Design review of the part shown in the three views and the two pictorial views. Dimensions are in mm from the part's minimum x, y and z. Give positions to 0.01 mm unless a question says otherwise; leave off trailing zeros. Loops run counter-clockwise (first coordinate to the right, second up) from the corner with the lowest first, then second, coordinate; pieces in that order, holes last. Notation, with made-up numbers: (-14.75, 44.25) -> (21.25, 44.25) arc R32 ccw to (21.25, 75.25) -> close; hole circle Ø9 at (-0.75, 79.25). An arc over 180 degrees is marked (long way). Answer as CSV lines item,"result".
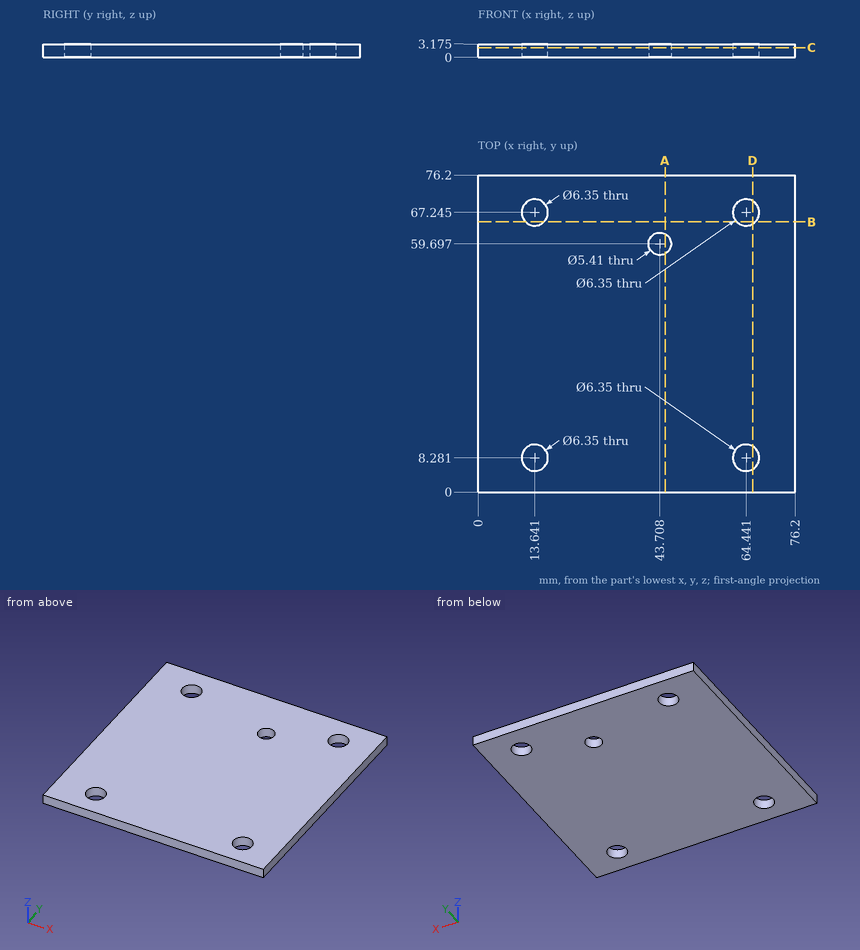
Q1. We need section D-D, the plane x = 66. State the section outline as (y, z) points (1 decimal).
Filled sheet:
outline,"(0, 0) -> (5.5, 0) -> (5.5, 3.2) -> (0, 3.2) -> close; (11, 0) -> (64.5, 0) -> (64.5, 3.2) -> (11, 3.2) -> close; (70, 0) -> (76.2, 0) -> (76.2, 3.2) -> (70, 3.2) -> close"
Q2. To check wall thickness, follow probe 1 along X at (y, z) = (67, 1.7) (1 decimal); probe 2 along Y at (x, z) = (67, 1.45) (1 decimal); probe 3 along X at (y, z) = (5.5, 2.8) (1 decimal). State the ranges of each line that lie inside material, in increasing order. Write a range as from..to.
Filled sheet:
probe 1,"x = 0..10.5, 16.8..61.3, 67.6..76.2"
probe 2,"y = 0..6.4, 10.2..65.4, 69.1..76.2"
probe 3,"x = 0..12.1, 15.2..62.9, 66..76.2"
Q3. We need section B-B, the plane y = 65. State the section outline as (x, z) points (1 decimal).
Filled sheet:
outline,"(0, 0) -> (11.4, 0) -> (11.4, 3.2) -> (0, 3.2) -> close; (15.9, 0) -> (62.2, 0) -> (62.2, 3.2) -> (15.9, 3.2) -> close; (66.7, 0) -> (76.2, 0) -> (76.2, 3.2) -> (66.7, 3.2) -> close"
Q4. Clearance check with a flat-ended pin moving along its axis: pin 1 Ø4 at (x, y) = (13.64, 8.28) entering from +Z. State where the tip first meets the part, or that it passes through.
Filled sheet:
pin 1,"passes through"
Q5. We need section A-A, the plane x = 45. State the section outline as (y, z) points (1 decimal).
Filled sheet:
outline,"(0, 0) -> (57.3, 0) -> (57.3, 3.2) -> (0, 3.2) -> close; (62.1, 0) -> (76.2, 0) -> (76.2, 3.2) -> (62.1, 3.2) -> close"
Q6. We need section C-C, the plane z = 2.3. State how many separate pieces and enclosed holes the cut face has, and give its area (3 significant figures).
Filled sheet:
separate pieces,"1"
enclosed holes,"5"
area,"5,660 mm^2"
